from build123d import *

# Parameters (mm, degrees)
F0_W     = 762
F0_H     = 609.6
F1_DEPTH = 19.05
F2_W     = 12.7
F2_H     = 12.8016
F3_DEPTH = 762.001
F4_W     = 12.7
F4_H     = 12.7
F5_DEPTH = 609.601


with BuildPart() as f1:
    # F0 (on Front) → F1 (new body)
    with BuildSketch(Plane.XZ):
        with Locations((381, 304.8)):
            Rectangle(F0_W, F0_H)
    extrude(amount=F1_DEPTH)

    # F2 (on face) → F3 (cut, through all)
    with BuildSketch(Plane.YZ.offset(762)):
        with Locations((-12.7, 6.4008)):
            Rectangle(F2_W, F2_H)
    extrude(amount=-F3_DEPTH, mode=Mode.SUBTRACT)

    # F4 (on face) → F5 (cut, through all)
    with BuildSketch(Plane.XY.offset(609.6)):
        with Locations((6.35, -12.7)):
            Rectangle(F4_W, F4_H)
    extrude(amount=-F5_DEPTH, mode=Mode.SUBTRACT)


solid = f1.part
Work out the finished part from the listing and answer in its coordinate system (mm). Give positions to 0.01 mm unless a question says otherwise; leave off trailing zeros. Order: outer loops, then holes, each group sorted by start corner. A loop starts at its lowest first (then second) coordinate and runs counter-clockwise, first axis right, second up. Notation, with made-up numbers: (66.25, 3) -> (95.25, 3) arc R14 ccw to (95.25, 28) -> close; hole circle Ø5 at (68, -17.5). An arc over 180 degrees is marked (long way). Answer as a JSON object with one key per item and string values. Group by question number.
1. A flat-ended cylindrical pin translates along its axis: pin 1 Ø5 at (x, y) = (136, -13.5) entering from -Z. Find the tip coordinate at first contact, or state that the pin passes through.
2. Section A-A on y = -10 is taken. Determine the outline of the cut face in (x, z), plus the area to 3 significant figures.
3. Consider line 1 along X through (y, z) = (-9.5, 497); line 2 along Z through (x, y) = (102.5, -13). Determine where each line is inside the solid, lowest interval first. Write a range as [from, to].
Result sheet:
{
 "1": {"pin 1": "stops at z = 12.8"},
 "2": {"outline": "(12.7, 12.8) -> (762, 12.8) -> (762, 609.6) -> (12.7, 609.6) -> close", "area": "447,000 mm^2"},
 "3": {"line 1": "x = [12.7, 762]", "line 2": "z = [12.8, 609.6]"}
}
